from build123d import *

# Parameters (mm, degrees)
F0_W     = 69.85
F0_H     = 50.8
F1_DEPTH = 50.8
F2_R     = 14.2875
F3_DEPTH = 50.801
F5_D     = 5.1054
F5_DEPTH = 25.4
F5_TIP   = 1.5338169022


with BuildPart() as f1:
    # F0 (on Front) → F1 (new body)
    with BuildSketch(Plane.XZ):
        with Locations((34.925, 25.4)):
            Rectangle(F0_W, F0_H)
    extrude(amount=F1_DEPTH)

    # F2 (on face) → F3 (cut, through all)
    with BuildSketch(Plane.XZ.offset(50.8)):
        with Locations((31.75, 25.4)):
            Circle(F2_R)
    extrude(amount=-F3_DEPTH, mode=Mode.SUBTRACT)

    # F5
    with Locations(Plane.YZ.offset(69.85)):
        with Locations((-25.4, 25.4)):
            Hole(F5_D / 2, depth=F5_DEPTH)
            with Locations((0, 0, -(F5_DEPTH + F5_TIP / 2))):  # 118° drill point
                Cone(0, F5_D / 2, F5_TIP, mode=Mode.SUBTRACT)


solid = f1.part
Design review of the part built by this model. Coordinates are the model's own, in mm. A direction names the side the tool comes from. Give positions to 0.01 mm unless a question says otherwise; leave off trailing zeros. Loops run counter-clockwise (first coordinate to the right, second up) from the corner with the lowest first, then second, coordinate; pieces in that order, holes last. Notation, with made-up numbers: (29, 54.5) - (60, 54.5) arc R17 ccw to (60, 65.5) - close; hole circle Ø8 at (41, 10). An arc over 180 degrees is marked (long way). Use CSV: the item, a comma, the result in double quotes. Start each with the question number.
1. Draft analysis for pull direction Z (two halves, no side actions). For faces 3 (the flat face through (34, -25, 0)), 4 (the flat face through (34, -25, 50.8)), 5 (the cylindrical face through (45.38, -25.76, 29.69)), 6 (the flat face through (0, -25, 25)), state which applies: released by +Z, released by -Z, zero draft, split by the parting line, or undercut.
2. Add section A-A (z = 25.4). State the section outline as (x, y) points, plus the area to 3 significant figures.
3. Machinability: for faces 1 (the flat face through (42, 0, 14)), 2 (the cylindrical face through (57.661, -26.772, 27.552)), which of the approach directions +Z, -Z, +X, -X, +Y, -Y give a long, thin tool a straight path to every point of the face, cutting with its end or side? Answer none if there is none.
4. Wall thickness on L1, parallel to Z at x = 63.5, y = -25.4; L2, parallel to X at y = -42, z = 25; L3, parallel to Y at x = 64.5, z = 25.4: over which ranges is each line inside the solid? List them lowest first.
5. Add section B-B (x = 31.75). State the section outline as (y, z) points.
6. Insertion check: P1, Ø3, axis at y = -27, z = 24.5, coming from the +X side. The pin has a flat end and moves straight along its axis. Give the tip position at first contact, or say it passes through.
7. Add section D-D (z = 36). State the section outline as (x, y) points.
Results found:
1,face 3,"released by -Z"
1,face 4,"released by +Z"
1,face 5,"undercut"
1,face 6,"zero draft"
2,outline,"(0, -50.8) - (17.46, -50.8) - (17.46, 0) - (0, 0) - close; (46.04, -50.8) - (69.85, -50.8) - (69.85, -27.95) - (46.04, -27.95) - close; (46.04, -22.85) - (69.85, -22.85) - (69.85, 0) - (46.04, 0) - close"
2,area,"1,980 mm²"
3,face 1,"+Z, -Z, +X, -X, +Y"
3,face 2,"+X"
4,L1,"z = 0 to 22.85, 27.95 to 50.8"
4,L2,"x = 0 to 17.47, 46.03 to 69.85"
4,L3,"y = -50.8 to -27.95, -22.85 to 0"
5,outline,"(-50.8, 0) - (0, 0) - (0, 11.11) - (-50.8, 11.11) - close; (-50.8, 39.69) - (0, 39.69) - (0, 50.8) - (-50.8, 50.8) - close"
6,P1,"stops at x = 69.85"
7,outline,"(0, -50.8) - (22.17, -50.8) - (22.17, 0) - (0, 0) - close; (41.33, -50.8) - (69.85, -50.8) - (69.85, 0) - (41.33, 0) - close"
